The listing builds one solid part. Answer for the finished solid, in the listing's coordinates (mm). A direction names the side the tool comes from. Give positions to 0.01 mm unless a question says otherwise; leave off trailing zeros. Order: outer loops, then holes, each group sorted by start corner. A loop starts at its lowest first (then second) coordinate and runs counter-clockwise, first axis right, second up. Notation, with made-up numbers: (8, 54.5) - (28, 54.5) arc R12 ccw to (28, 77.5) - close; hole circle Ø4 at (-12, 22). An arc over 180 degrees is marked (long way). Write each question's results on one line, items separated by ' | '. Start each with the question number.
1. A flat-ended cylindrical pin translates along its axis: pin 1 (5 mm diameter, centred on x = -22, y = 28, fed in from -Z). Find the tip coordinate at first contact, or state that the pin passes through.
2. Which of the six approach directions +Z, -Z, +X, -X, +Y, -Y give full straight-line access (tool end or side, diameter ignored) to faces 1 (the face through (29.1, 1, -1)), 2 (the face through (0.228, -31.265, 0.986))?
3. Section A-A (x = 0) is taken. Give the vertices of the cut face in (y, z).
4. Find the intervals of material crossed by L1, parallel to Y at x = 0, z = 0.95; L2, parallel to X at y = -13, z = -0.1; L3, parallel to Z at x = 14.5, y = -12.5, in increasing order.
5. Section C-C (z = -0.8) is taken. Give the vertices of the cut face in (x, y).
6. Section D-D (y = 24) is taken. Give the vertices of the cut face in (x, z), and give its area (3 significant figures).
7. Determine the mould class of faces 3 (the face through (0, 1, 2)), 4 (the face through (30.4, 0.55, 1.43)), 5 (the face through (-30.4, -0.55, 1.43)), 6 (the face through (-29.1, 0, -1)) for opening direction X: released by +X, released by -X, zero draft, split by the parting line, or undercut.
8. Section B-B (y = -33) is taken. Give the vertices of the cut face in (x, z).
Autodesk Inventor part; units mm, degrees
ref_plane "YZ Plane" through (0, 0, 0) normal (1, 0, 0) x (0, 1, 0)
ref_plane "XZ Plane" through (0, 0, 0) normal (0, 1, 0) x (-1, 0, 0)
ref_plane "XY Plane" through (0, 0, 0) normal (0, 0, 1) x (1, 0, 0)
sketch "스케치1" plane through (0, 0, 0) normal (0, 0, 1) x (1, 0, 0)
  line L0 (-31, -39) -> (31, -39)
  line L1 (31, -39) -> (31, 39)
  line L2 (31, 39) -> (-31, 39)
  line L3 (-31, 39) -> (-31, -39)
  line L4 (-31, -39) -> (31, 39) construction
  line L5 (31, -39) -> (-31, 39) construction
  line L6 (-29.1, 37.1) -> (29.1, 37.1)
  line L7 (29.1, 37.1) -> (29.1, -37.1)
  line L8 (29.1, -37.1) -> (-29.1, -37.1)
  line L9 (-29.1, -37.1) -> (-29.1, 37.1)
  line L10 (-29.1, 37.1) -> (-29.1, 39)
  line L11 (29.1, 37.1) -> (29.1, 39)
  point P0 (0, 0)
  dimension "d0" = 62
  dimension "d1" = 78
  dimension "d2" = 1.9
extrude "돌출1" add sketch "스케치1" against normal blind 2 contours L3 L2 L10 L9 L8 L7 L11 L1 L0
extrude "돌출2" add sketch "스케치1" along normal blind 2
sketch "스케치2" plane through (0, 0, 0) normal (0, 0, -1) x (-1, 0, 0)
  line L0 (-3, -45) -> (3, -45)
  line L1 (3, -45) -> (3, -33)
  line L2 (3, -33) -> (-3, -33) construction
  line L3 (-3, -33) -> (-3, -45)
  line L4 (31, -39) -> (-31, -39)
  line L5 (-3, -45) -> (3, -33) construction
  line L6 (3, -45) -> (-3, -33) construction
  circle A0 centre (0, -33) radius 3
  circle A1 centre (0, -33) radius 1.75
  point P0 (0, 0)
  point P1 (0, -39)
  point P2 (-3, -39)
  point P3 (3, -39)
  dimension "d7" = 12
  dimension "d8" = 6
  dimension "d9" = 3.5
extrude "돌출4" cut sketch "스케치2" against normal blind 2 contours A1
fillet "모깎기1" radius 2 2 edges at (-31, 0, 2) (31, 0, 2)
properties part number "커튼 정면 커버"
Reported:
1) pin 1: z = 0
2) face 1: -Z, +Y | face 2: +Z, -Z
3) outline: (-39, -2) - (-37.1, -2) - (-37.1, 0) - (-34.75, 0) - (-34.75, 2) - (-39, 2) - close; (-31.25, 0) - (39, 0) - (39, 2) - (-31.25, 2) - close
4) L1: -39 to -34.75, -31.25 to 39 | L2: -31 to -29.1, 29.1 to 31 | L3: 0 to 2
5) outline: (-31, -39) - (31, -39) - (31, 39) - (29.1, 39) - (29.1, -37.1) - (-29.1, -37.1) - (-29.1, 39) - (-31, 39) - close
6) outline: (-31, -2) - (-29.1, -2) - (-29.1, 0) - (29.1, 0) - (29.1, -2) - (31, -2) - (31, 0) arc R2 ccw to (29, 2) - (-29, 2) arc R2 ccw to (-31, 0) - close | area: 130 mm²
7) face 3: zero draft | face 4: released by +X | face 5: released by -X | face 6: undercut
8) outline: (-31, -2) - (-29.1, -2) - (-29.1, 0) - (-1.75, 0) - (-1.75, 2) - (-29, 2) arc R2 ccw to (-31, 0) - close; (1.75, 0) - (29.1, 0) - (29.1, -2) - (31, -2) - (31, 0) arc R2 ccw to (29, 2) - (1.75, 2) - close
